Autodesk Inventor part; units mm, degrees
ref_plane "YZ Plane" through (0, 0, 0) normal (1, 0, 0) x (0, 1, 0)
ref_plane "XZ Plane" through (0, 0, 0) normal (0, 1, 0) x (-1, 0, 0)
ref_plane "XY Plane" through (0, 0, 0) normal (0, 0, 1) x (1, 0, 0)
sketch "Sketch1" plane through (0, 0, 0) normal (0, 1, 0) x (-1, 0, 0)
  line L0 (0, 0) -> (60, 0)
  line L1 (60, 0) -> (60, -10)
  line L2 (60, -10) -> (0, -10)
  line L3 (0, -10) -> (0, 0)
  circle A0 centre (4, -5) radius 1
  circle A1 centre (56, -5) radius 1
  line L4 (60, -5) -> (0, -5) construction
  dimension "d0" = 10
  dimension "d1" = 60
  dimension "d2" = 2
  dimension "d3" = 4
  dimension "d4" = 4
extrude "Extrusion1" add sketch "Sketch1" along normal blind 6
fillet "Fillet1" radius 4 2 edges at (0, 3, -10) (-60, 3, -10)
properties part number "humidity_support"
Could you check a few things on this model? Use its own coordinates, in mm. Give positions to 0.01 mm unless a question says otherwise; leave off trailing zeros. Order: outer loops, then holes, each group sorted by start corner. A loop starts at its lowest first (then second) coordinate and runs counter-clockwise, first axis right, second up. Notation, with made-up numbers: (46.5, 56.5) - (97.5, 56.5) arc R14 cw to (97.5, 72.5) - close; hole circle Ø6 at (37.5, -30). An arc over 180 degrees is marked (long way). One line per item, written item: value. Start each with the question number.
1. If I drill on probe 1 along Z at (x, y) = (-4, 1.6); probe 2 along X at (y, z) = (4.1, -5.5); probe 3 along Z at (x, y) = (-4.5, 2.35), over which ranges is the centre line in solid material (lowest first)?
2. Imagine slicing it at B-B on z = -5. List the corners of the cut face in (x, y) for me, plus the area to 3 significant figures.
3. Imagine slicing it at C-C on z = -8. List the corners of the cut face in (x, y) for me.
4. For P1, Ø1.5, axis at y = 2, z = -7, coming from the -X side, with a flat end and sliding along its axis, tell me the tip position at first contact or that it passes through.
5. Thinking about a two-plate mould opening in Z: for faces 1 (the face through (-58.797, 3.042, -8.859)), 2 (the face through (-55, 3, -5)), 3 (the face through (-60, 3, -3)), 4 (the face through (-30, 3, 0)), which applies, +Z half, -Z half, draft (parallel to the pull), parting line (faces both ways), or undercut?
6. Imagine slicing it at A-A on y = 2.5. List the corners of the cut face in (x, z) for me.
Values:
1. probe 1: -10 to -6, -4 to 0
1. probe 2: -60 to -56.87, -55.13 to -4.87, -3.13 to 0
1. probe 3: -10 to -5.87, -4.13 to 0
2. outline: (-60, 0) - (-57, 0) - (-57, 6) - (-60, 6) - close; (-55, 0) - (-5, 0) - (-5, 6) - (-55, 6) - close; (-3, 0) - (0, 0) - (0, 6) - (-3, 6) - close
2. area: 336 mm²
3. outline: (-59.46, 0) - (-0.54, 0) - (-0.54, 6) - (-59.46, 6) - close
4. P1: x = -59.99
5. face 1: -Z half
5. face 2: undercut
5. face 3: draft
5. face 4: +Z half
6. outline: (-60, -6) arc R4 ccw to (-56, -10) - (-4, -10) arc R4 ccw to (0, -6) - (0, 0) - (-60, 0) - close; hole circle Ø2 at (-56, -5); hole circle Ø2 at (-4, -5)
